Input: part model. Units: mm. Frame: model coordinates. Give positions to 0.01 mm unless a question says otherwise; leave off trailing zeros. Write each loop counter-clockwise with the first axis right and the second up, starting at its lowest first coordinate (ties: lowest second). Pieces come first, ordered by that corner, then holes. Notation, with made-up numbers: (24, 32.5) - (66, 32.5) arc R31 cw to (66, 67.5) - close; hole circle Ø2 at (-14, 29.5). An arc over 180 degrees is marked (long way). Use a Markdown table: item, result. Add a question column.
1. Section query A-A, the plane y = 130.5. Return loops of the section in (x, z).
2. Section query C-C, the plane z = 24.5. Count the separate pieces of the cut face and the enclosed holes in it, plus the area to 3 significant figures.
3. Section query D-D, the plane y = 151. Return loops of the section in (x, z).
4. Material intervals for probe 1 along Y at (x, z) = (-5.5, 18); probe 2 along Y at (x, z) = (30.5, 16.5); probe 3 along X at (y, z) = (74, 30.5), sorted ascending.
5. Section query B-B, the plane x = 11.5. Return loops of the section in (y, z), plus the area to 3 significant figures.
6. Mould query, pull axis X, two halves, no side actions, for faces 1 (the flat face through (-15.181, 53, 17)), 2 (the flat face through (23, 167.274, 17)), 3 (the flat face through (22.819, 80, 19)). Classes: released by +X, released by -X, zero draft, split by the parting line, or undercut.
```python
from build123d import *

# Parameters (mm, degrees)
F2_W      = 2
F2_H      = 110
F3_DEPTH  = 4
F4_W      = 2
F4_H      = 33
F4_H_2    = 40
F4_H_3    = 27
F4_H_4    = 19
F4_H_5    = 35
F4_W_2    = 7
F4_H_6    = 2
F5_DEPTH  = 30
F6_W      = 12
F6_H      = 25
F6_W_2    = 27
F7_DEPTH  = 2
F8_W      = 12
F8_H      = 25
F8_W_2    = 20
F8_H_2    = 13
F9_DEPTH  = 2
F10_W     = 22
F10_H     = 19
F11_DEPTH = 2
F12_W     = 12
F12_H     = 25
F12_W_2   = 10.6349699199
F13_DEPTH = 2


with BuildPart() as f3:
    # F2 (on Top) → F3 (new body)
    with BuildSketch(Plane.XY):
        Polygon((57.8188975325, 167.2736013268), (-13.1811024675, 167.2736013268), (-13.1811024675, 107.2736013268), (-13.1811024675, -2.7263986732), (57.8188975325, -2.7263986732), align=None)
        with Locations((-14.1811024675, 52.2736013268)):
            Rectangle(F2_W, F2_H)
    extrude(amount=F3_DEPTH)

    # F4 (on face) → F5 (join)
    with BuildSketch(Plane.XY.offset(4)):
        with Locations((56.8188975325, 15.7736013268)):
            Rectangle(F4_W, F4_H)
        with Locations((56.8188975325, 54.2736013268)):
            Rectangle(F4_W, F4_H_2)
        Polygon((-13.1811024675, 167.2736013268), (-13.1811024675, 107.2736013268), (-11.1811024675, 107.2736013268), (-11.1811024675, 165.2736013268), (-11.1811024675, 167.2736013268), align=None)
        Polygon((-11.1811024675, 167.2736013268), (-11.1811024675, 165.2736013268), (55.8188975325, 165.2736013268), (57.8188975325, 165.2736013268), (57.8188975325, 167.2736013268), align=None)
        Polygon((-15.1811024675, -0.7263986732), (-15.1811024675, -2.7263986732), (57.8188975325, -2.7263986732), (57.8188975325, -0.7263986732), (55.8188975325, -0.7263986732), (27.8188975325, -0.7263986732), (25.8188975325, -0.7263986732), (-13.1811024675, -0.7263986732), align=None)
        Polygon((-11.1811024675, 107.2736013268), (-13.1811024675, 107.2736013268), (-13.1811024675, 105.2736013268), (20.8188975325, 105.2736013268), (22.8188975325, 105.2736013268), (22.8188975325, 107.2736013268), align=None)
        Polygon((55.8188975325, 76.2736013268), (57.8188975325, 76.2736013268), (57.8188975325, 165.2736013268), (55.8188975325, 165.2736013268), (55.8188975325, 97.2736013268), (55.8188975325, 95.2736013268), align=None)
        Polygon((-15.1811024675, 107.2736013268), (-15.1811024675, -0.7263986732), (-13.1811024675, -0.7263986732), (-13.1811024675, 32.2736013268), (-13.1811024675, 34.2736013268), (-13.1811024675, 76.2736013268), (-13.1811024675, 78.2736013268), (-13.1811024675, 105.2736013268), (-13.1811024675, 107.2736013268), align=None)
        Polygon((55.8188975325, 74.2736013268), (57.8188975325, 74.2736013268), (57.8188975325, 76.2736013268), (55.8188975325, 76.2736013268), (31.8188975325, 76.2736013268), (29.8188975325, 76.2736013268), (29.8188975325, 74.2736013268), (31.8188975325, 74.2736013268), align=None)
        Polygon((55.8188975325, 32.2736013268), (57.8188975325, 32.2736013268), (57.8188975325, 34.2736013268), (55.8188975325, 34.2736013268), (31.8188975325, 34.2736013268), (29.8188975325, 34.2736013268), (22.8188975325, 34.2736013268), (20.8188975325, 34.2736013268), (-13.1811024675, 34.2736013268), (-13.1811024675, 32.2736013268), (25.8188975325, 32.2736013268), (27.8188975325, 32.2736013268), align=None)
        with Locations((21.8188975325, 91.7736013268)):
            Rectangle(F4_W, F4_H_3)
        Polygon((20.8188975325, 76.2736013268), (20.8188975325, 34.2736013268), (22.8188975325, 34.2736013268), (22.8188975325, 52.2736013268), (22.8188975325, 54.2736013268), (22.8188975325, 76.2736013268), align=None)
        Polygon((-13.1811024675, 78.2736013268), (-13.1811024675, 76.2736013268), (20.8188975325, 76.2736013268), (22.8188975325, 76.2736013268), (22.8188975325, 78.2736013268), (20.8188975325, 78.2736013268), align=None)
        with Locations((30.8188975325, 85.7736013268)):
            Rectangle(F4_W, F4_H_4)
        Polygon((55.8188975325, 95.2736013268), (55.8188975325, 97.2736013268), (31.8188975325, 97.2736013268), (29.8188975325, 97.2736013268), (29.8188975325, 95.2736013268), (31.8188975325, 95.2736013268), align=None)
        with Locations((30.8188975325, 114.7736013268)):
            Rectangle(F4_W, F4_H_5)
        Polygon((29.8188975325, 34.2736013268), (31.8188975325, 34.2736013268), (31.8188975325, 74.2736013268), (29.8188975325, 74.2736013268), (29.8188975325, 54.2736013268), (29.8188975325, 52.2736013268), align=None)
        with Locations((26.3188975325, 53.2736013268)):
            Rectangle(F4_W_2, F4_H_6)
    extrude(amount=F5_DEPTH)

    # F6 (on face) → F7 (cut)
    with BuildSketch(Plane(origin=(-13.1811024675, 0, 0), x_dir=(0, -1, 0), z_dir=(-1, 0, 0))):
        with Locations((-118.2736013268, 16.5)):
            Rectangle(F6_W, F6_H)
        with Locations((-145.7736013268, 16.5)):
            Rectangle(F6_W_2, F6_H)
    extrude(amount=-F7_DEPTH, mode=Mode.SUBTRACT)

    # F8 (on face) → F9 (cut)
    with BuildSketch(Plane(origin=(55.8188975325, 0, 0), x_dir=(0, -1, 0), z_dir=(-1, 0, 0))):
        with Locations((-113.2736013268, 16.5)):
            Rectangle(F8_W, F8_H)
        with Locations((-133.2736013268, 22.5)):
            Rectangle(F8_W_2, F8_H_2)
    extrude(amount=-F9_DEPTH, mode=Mode.SUBTRACT)

    # F10 (on face) → F11 (cut)
    with BuildSketch(Plane.XZ.offset(-165.2736013268)):
        with Locations((42.8188975325, 19.5)):
            Rectangle(F10_W, F10_H)
        with Locations((7.8188975325, 19.5)):
            Rectangle(F10_W, F10_H)
    extrude(amount=-F11_DEPTH, mode=Mode.SUBTRACT)

    # F12 (on face) → F13 (cut)
    with BuildSketch(Plane(origin=(20.8188975325, 0, 0), x_dir=(0, -1, 0), z_dir=(-1, 0, 0))):
        with Locations((-87.2736013268, 16.5)):
            Rectangle(F12_W, F12_H)
        with Locations((-62.9561163669, 16.5)):
            Rectangle(F12_W_2, F12_H)
        with Locations((-45.2736013268, 16.5)):
            Rectangle(F12_W, F12_H)
    extrude(amount=-F13_DEPTH, mode=Mode.SUBTRACT)


solid = f3.part
```
Result sheet:
| question | item | result |
|---|---|---|
| 1 | outline | (-13.18, 0) - (57.82, 0) - (57.82, 16) - (55.82, 16) - (55.82, 4) - (31.82, 4) - (31.82, 34) - (29.82, 34) - (29.82, 4) - (-11.18, 4) - (-11.18, 34) - (-13.18, 34) - close; (55.82, 29) - (57.82, 29) - (57.82, 34) - (55.82, 34) - close |
| 2 | separate pieces | 6 |
| 2 | enclosed holes | 3 |
| 2 | area | 1,380 mm² |
| 3 | outline | (-13.18, 0) - (57.82, 0) - (57.82, 34) - (55.82, 34) - (55.82, 4) - (-13.18, 4) - close; (-13.18, 29) - (-11.18, 29) - (-11.18, 34) - (-13.18, 34) - close |
| 4 | probe 1 | y = -2.73 to -0.73, 32.27 to 34.27, 76.27 to 78.27, 105.27 to 107.27, 165.27 to 167.27 |
| 4 | probe 2 | y = -2.73 to -0.73, 32.27 to 132.27, 165.27 to 167.27 |
| 4 | probe 3 | x = -15.18 to -13.18, 20.82 to 22.82, 29.82 to 31.82, 55.82 to 57.82 |
| 5 | outline | (-2.73, 0) - (167.27, 0) - (167.27, 10) - (165.27, 10) - (165.27, 4) - (107.27, 4) - (107.27, 34) - (105.27, 34) - (105.27, 4) - (78.27, 4) - (78.27, 34) - (76.27, 34) - (76.27, 4) - (34.27, 4) - (34.27, 34) - (32.27, 34) - (32.27, 4) - (-0.73, 4) - (-0.73, 34) - (-2.73, 34) - close; (165.27, 29) - (167.27, 29) - (167.27, 34) - (165.27, 34) - close |
| 5 | area | 942 mm² |
| 6 | face 1 | released by -X |
| 6 | face 2 | zero draft |
| 6 | face 3 | undercut |
